Read the model definition and answer for the solid it produces. Units are mm, in the model's axes. A direction names the side the tool comes from. Coordinates: 2 decimals unless noted, no trailing zeros. Order: outer loops, then holes, each group sorted by start corner. A loop starts at its lowest first (then second) coordinate and runs counter-clockwise, first axis right, second up.
Autodesk Inventor part; units mm, degrees
ref_plane "YZ Plane" through (0, 0, 0) normal (1, 0, 0) x (0, 1, 0)
ref_plane "XZ Plane" through (0, 0, 0) normal (0, 1, 0) x (-1, 0, 0)
ref_plane "XY Plane" through (0, 0, 0) normal (0, 0, 1) x (1, 0, 0)
sketch "Boceto1" plane through (0, 0, 0) normal (0, 1, 0) x (-1, 0, 0)
  circle A0 centre (0, 0) radius 3.15
  line L0 (6.889, 30) -> (3.889, 30)
  line L1 (3.889, -30) -> (6.889, -30)
  line L2 (6.889, -30) -> (6.889, 30)
  line L3 (0, 0) -> (3.15, 0) construction
  arc A1 (0, 6.889) -> (0, -6.889) centre (0, 0) ccw
  line L4 (3.889, 30) -> (3.889, 10.7779)
  line L5 (3.889, -30) -> (3.889, -10.7779)
  arc A2 (0, 6.889) -> (3.889, 10.7779) centre (0, 10.7779) ccw
  arc A3 (3.889, -10.7779) -> (0, -6.889) centre (0, -10.7779) ccw
  line L6 (2.9445, 5.1) -> (5.889, 0) construction
  line L7 (5.889, 0) -> (2.9445, -5.1) construction
  line L8 (2.9445, -5.1) -> (-2.9445, -5.1) construction
  line L9 (-2.9445, -5.1) -> (-5.889, 0) construction
  line L10 (-5.889, 0) -> (-2.9445, 5.1) construction
  line L11 (-2.9445, 5.1) -> (2.9445, 5.1) construction
  line L12 (5.889, 0) -> (6.889, 0) construction
  line L13 (-5.889, 0) -> (-6.889, 0) construction
  line L14 (0, -10.7779) -> (0, 0) construction
  dimension "d0" = 6.3
  dimension "d3" = 10.2
  dimension "d4" = 1
  dimension "d5" = 3
  dimension "d12" = 60
extrude "Extrusión1" add sketch "Boceto1" along normal blind 70
sketch "Boceto2" plane through (0, 0, 0) normal (0, -1, 0) x (1, 0, 0)
  line L0 (-5.7735, 0) -> (-2.8868, 5)
  line L1 (-2.8868, 5) -> (2.8868, 5)
  line L2 (2.8868, 5) -> (5.7735, 0)
  line L3 (5.7735, 0) -> (2.8868, -5)
  line L4 (2.8868, -5) -> (-2.8868, -5)
  line L5 (-2.8868, -5) -> (-5.7735, 0)
  point P0 (0, 0)
  point P1 (0, 0)
  dimension "d8" = 10
extrude "Extrusión2" cut sketch "Boceto2" against normal blind 6
sketch "Boceto4" plane through (-6.889, 0, -30) normal (-1, 0, 0) x (0, 0, 1)
  line L0 (10.7549, 2) -> (15.7549, 2)
  line L1 (15.7549, 2) -> (15.7549, 0)
  line L2 (15.7549, 0) -> (10.7549, 0)
  line L3 (10.7549, 0) -> (10.7549, 2)
  line L4 (44.2451, 2) -> (49.2451, 2)
  line L5 (49.2451, 2) -> (49.2451, 0)
  line L6 (49.2451, 0) -> (44.2451, 0)
  line L7 (44.2451, 0) -> (44.2451, 2)
  line L8 (0, 0) -> (60, 0)
  line L9 (30, 0) -> (30, 6)
  line L10 (30, 0) -> (30, 70) construction
  line L11 (0, 70) -> (60, 70)
  line L12 (30, 35) -> (1.5097, 35) construction
  line L13 (10.7549, 68) -> (15.7549, 68)
  line L14 (15.7549, 68) -> (15.7549, 70)
  line L15 (15.7549, 70) -> (10.7549, 70)
  line L16 (10.7549, 70) -> (10.7549, 68)
  line L17 (44.2451, 68) -> (49.2451, 68)
  line L18 (49.2451, 68) -> (49.2451, 70)
  line L19 (49.2451, 70) -> (44.2451, 70)
  line L20 (44.2451, 70) -> (44.2451, 68)
  point P0 (47.493, 22.347)
  dimension "d19" = 5
  dimension "d20" = 2
extrude "Extrusión3" cut sketch "Boceto4" against normal up to next
fillet "Empalme1" radius 5 4 edges at (-5.389, 70, -30) (-5.389, 70, 30) (-5.389, 0, 30) (-5.389, 0, -30)
properties part number "Soporte ESC"
1) A cutting plane is placed at B-B, the plane x = 0.75. Determine the outline of the cut face in (y, z), and give its area (3 significant figures).
A:
outline: (0, -6.85) - (70, -6.85) - (70, -3.06) - (6, -3.06) - (6, -5) - (0, -5) - close; (0, 5) - (6, 5) - (6, 3.06) - (70, 3.06) - (70, 6.85) - (0, 6.85) - close
area: 507 mm2
2) Which of the six approach directions +Z, -Z, +X, -X, +Y, -Y give full straight-line access (tool end or side, diameter ignored) to faces 1 (the flat face through (-5, 69, -14.245)), 2 (the flat face through (-5, 1, -14.245)), 3 (the cylindrical face through (-5, 69, -28)), 4 (the flat face through (-3.889, 35, -21)), 5 (the flat face through (2.5, 6, 2.3))?
A:
face 1: +X, -X, +Y
face 2: +X, -X, -Y
face 3: -Z, +X, -X, +Y
face 4: -Z, +X, +Y, -Y
face 5: -Y
3) Flat-ended cylindrical pins translate along their axes: pin 1 Ø1.5 at (x, z) = (-5.5, 17) entering from +Y; pin 2 Ø1.6 at (x, y) = (-5, 1) entering from -Z; pin 3 Ø0.6 at (x, y) = (-5.5, 69) entering from +Z; pin 4 Ø5 at (x, z) = (0, 0) entering from +Y. Find the tip coordinate at first contact, or state that the pin passes through.
A:
pin 1: stops at y = 68
pin 2: stops at z = -28.84
pin 3: stops at z = 28.36
pin 4: passes through
4) A cutting plane is placed at A-A, the plane y = 22.5. Determine the outline of the cut face in (x, z).
A:
outline: (-6.89, -30) - (-3.89, -30) - (-3.89, -10.78) arc R3.89 cw to (0, -6.89) arc R6.89 ccw to (0, 6.89) arc R3.89 cw to (-3.89, 10.78) - (-3.89, 30) - (-6.89, 30) - close; hole circle Ø6.3 at (0, 0)
5) Determine the mould class of faces 6 (the flat face through (-5, 68, 17)), 7 (the cylindrical face through (2.5, 37.552, 1.917)), 8 (the cylindrical face through (6.887, 34.51, -0.151)), 9 (the flat face through (-4.31, 2.958, -2.535)) for opening direction X: pulls with the +X half, pulls with the -X half, needs draft (parallel to the pull), parting line crosses it, or undercut.
A:
face 6: needs draft
face 7: undercut
face 8: pulls with the +X half
face 9: undercut
6) A cutting plane is placed at C-C, the plane z = 20. Determine the outline of the cut face in (x, y), and give its area (3 significant figures).
A:
outline: (-6.89, 0) - (-3.89, 0) - (-3.89, 70) - (-6.89, 70) - close
area: 210 mm2
7) Straight lines are drawn through the part: line 1 (Z direction, x = 0, y = 39); line 2 (X direction, y = 47.5, z = -22.5). For each, find the intervals that lie inside material, in ascending order.
A:
line 1: z = -6.89 to -3.15, 3.15 to 6.89
line 2: x = -6.89 to -3.89
8) A cutting plane is placed at D-D, the plane z = -9.5. Determine the outline of the cut face in (x, y), and give its area (3 significant figures).
A:
outline: (-6.89, 0) - (-3.67, 0) - (-3.67, 70) - (-6.89, 70) - close
area: 225 mm2
